```python
from build123d import *

# Parameters (mm, degrees)
SKETCH1_W           = 150
SKETCH1_H           = 150
SKETCH1_R           = 3
BOSS_EXTRUDE1_DEPTH = 60
SKETCH4_R           = 10
BOSS_EXTRUDE3_DEPTH = 8
SKETCH4_6_R         = 10
CUT_EXTRUDE1_DEPTH  = 5
SKETCH5_R           = 10
CUT_EXTRUDE2_DEPTH  = 5
SKETCH6_R           = 10
BOSS_EXTRUDE4_DEPTH = 5
SKETCH7_R           = 10
BOSS_EXTRUDE5_DEPTH = 5
CUT_EXTRUDE3_DEPTH  = 15


with BuildPart() as part:
    # Sketch1 → Boss-Extrude1 (new body)
    with BuildSketch(Plane(origin=(0, 0, 0), x_dir=(1, 0, 0), z_dir=(0, 1, 0))):
        with Locations((19.022617124, 32.835218094)):
            Rectangle(SKETCH1_W, SKETCH1_H)
        with Locations(Location((-43.477382875, 95.335218094, 0), (0, 0, 270))):
            Circle(SKETCH1_R, mode=Mode.SUBTRACT)
        with Locations(Location((-18.477382875, 95.335218094, 0), (0, 0, 270))):
            Circle(SKETCH1_R, mode=Mode.SUBTRACT)
        with Locations(Location((6.522617125, 95.335218094, 0), (0, 0, 270))):
            Circle(SKETCH1_R, mode=Mode.SUBTRACT)
        with Locations(Location((31.522617125, 95.335218094, 0), (0, 0, 270))):
            Circle(SKETCH1_R, mode=Mode.SUBTRACT)
        with Locations(Location((56.522617125, 95.335218094, 0), (0, 0, 270))):
            Circle(SKETCH1_R, mode=Mode.SUBTRACT)
        with Locations(Location((81.522617125, 95.335218094, 0), (0, 0, 270))):
            Circle(SKETCH1_R, mode=Mode.SUBTRACT)
        with Locations(Location((-18.477382875, 70.335218094, 0), (0, 0, 270))):
            Circle(SKETCH1_R, mode=Mode.SUBTRACT)
        with Locations(Location((6.522617125, 70.335218094, 0), (0, 0, 270))):
            Circle(SKETCH1_R, mode=Mode.SUBTRACT)
        with Locations(Location((31.522617125, 70.335218094, 0), (0, 0, 270))):
            Circle(SKETCH1_R, mode=Mode.SUBTRACT)
        with Locations(Location((56.522617125, 70.335218094, 0), (0, 0, 270))):
            Circle(SKETCH1_R, mode=Mode.SUBTRACT)
        with Locations(Location((81.522617125, 70.335218094, 0), (0, 0, 270))):
            Circle(SKETCH1_R, mode=Mode.SUBTRACT)
        with Locations(Location((-18.477382875, 45.335218094, 0), (0, 0, 270))):
            Circle(SKETCH1_R, mode=Mode.SUBTRACT)
        with Locations(Location((6.522617125, 45.335218094, 0), (0, 0, 270))):
            Circle(SKETCH1_R, mode=Mode.SUBTRACT)
        with Locations(Location((31.522617125, 45.335218094, 0), (0, 0, 270))):
            Circle(SKETCH1_R, mode=Mode.SUBTRACT)
        with Locations(Location((56.522617125, 45.335218094, 0), (0, 0, 270))):
            Circle(SKETCH1_R, mode=Mode.SUBTRACT)
        with Locations(Location((81.522617125, 45.335218094, 0), (0, 0, 270))):
            Circle(SKETCH1_R, mode=Mode.SUBTRACT)
        with Locations(Location((-18.477382875, 20.335218094, 0), (0, 0, 270))):
            Circle(SKETCH1_R, mode=Mode.SUBTRACT)
        with Locations(Location((6.522617125, 20.335218094, 0), (0, 0, 270))):
            Circle(SKETCH1_R, mode=Mode.SUBTRACT)
        with Locations(Location((31.522617125, 20.335218094, 0), (0, 0, 270))):
            Circle(SKETCH1_R, mode=Mode.SUBTRACT)
        with Locations(Location((56.522617125, 20.335218094, 0), (0, 0, 270))):
            Circle(SKETCH1_R, mode=Mode.SUBTRACT)
        with Locations(Location((81.522617125, 20.335218094, 0), (0, 0, 270))):
            Circle(SKETCH1_R, mode=Mode.SUBTRACT)
        with Locations(Location((-18.477382875, -4.664781906, 0), (0, 0, 270))):
            Circle(SKETCH1_R, mode=Mode.SUBTRACT)
        with Locations(Location((6.522617125, -4.664781906, 0), (0, 0, 270))):
            Circle(SKETCH1_R, mode=Mode.SUBTRACT)
        with Locations(Location((31.522617125, -4.664781906, 0), (0, 0, 270))):
            Circle(SKETCH1_R, mode=Mode.SUBTRACT)
        with Locations(Location((56.522617125, -4.664781906, 0), (0, 0, 270))):
            Circle(SKETCH1_R, mode=Mode.SUBTRACT)
        with Locations(Location((81.522617125, -4.664781906, 0), (0, 0, 270))):
            Circle(SKETCH1_R, mode=Mode.SUBTRACT)
        with Locations(Location((-18.477382875, -29.664781906, 0), (0, 0, 270))):
            Circle(SKETCH1_R, mode=Mode.SUBTRACT)
        with Locations(Location((6.522617125, -29.664781906, 0), (0, 0, 270))):
            Circle(SKETCH1_R, mode=Mode.SUBTRACT)
        with Locations(Location((31.522617125, -29.664781906, 0), (0, 0, 270))):
            Circle(SKETCH1_R, mode=Mode.SUBTRACT)
        with Locations(Location((56.522617125, -29.664781906, 0), (0, 0, 270))):
            Circle(SKETCH1_R, mode=Mode.SUBTRACT)
        with Locations(Location((81.522617125, -29.664781906, 0), (0, 0, 270))):
            Circle(SKETCH1_R, mode=Mode.SUBTRACT)
        with Locations(Location((-43.477382875, 70.335218094, 0), (0, 0, 270))):
            Circle(SKETCH1_R, mode=Mode.SUBTRACT)
        with Locations(Location((-43.477382875, 45.335218094, 0), (0, 0, 270))):
            Circle(SKETCH1_R, mode=Mode.SUBTRACT)
        with Locations(Location((-43.477382875, 20.335218094, 0), (0, 0, 270))):
            Circle(SKETCH1_R, mode=Mode.SUBTRACT)
        with Locations(Location((-43.477382875, -4.664781906, 0), (0, 0, 270))):
            Circle(SKETCH1_R, mode=Mode.SUBTRACT)
        with Locations(Location((-43.477382875, -29.664781906, 0), (0, 0, 270))):
            Circle(SKETCH1_R, mode=Mode.SUBTRACT)
    extrude(amount=BOSS_EXTRUDE1_DEPTH)

    # Sketch4 → Boss-Extrude3 (add)
    with BuildSketch(Plane(origin=(94.022617124, 0, 0), x_dir=(0, 0, -1), z_dir=(1, 0, 0))):
        with Locations((57.835218094, 30)):
            Circle(SKETCH4_R)
    extrude(amount=-BOSS_EXTRUDE3_DEPTH)

    # Sketch4_6 → Cut-Extrude1 (cut)
    with BuildSketch(Plane(origin=(94.022617124, 0, 0), x_dir=(0, 0, -1), z_dir=(1, 0, 0))):
        with Locations((7.835218094, 30)):
            Circle(SKETCH4_6_R)
        with Locations((57.835218094, 30)):
            Circle(SKETCH4_6_R)
    extrude(amount=-CUT_EXTRUDE1_DEPTH, mode=Mode.SUBTRACT)

    # Sketch5 → Cut-Extrude2 (cut)
    with BuildSketch(Plane(origin=(0, 0, -107.835218094), x_dir=(-1, 0, 0), z_dir=(0, 0, -1))):
        with Locations((-44.022617124, 30)):
            Circle(SKETCH5_R)
        with Locations((5.977382876, 30)):
            Circle(SKETCH5_R)
    extrude(amount=-CUT_EXTRUDE2_DEPTH, mode=Mode.SUBTRACT)

    # Sketch6 → Boss-Extrude4 (add)
    with BuildSketch(Plane.ZY.offset(55.977382876)):
        with Locations(Location((-57.835218094, 30, 0), (0, 0, 180))):
            Circle(SKETCH6_R)
        with Locations(Location((-7.835218094, 30, 0), (0, 0, 180))):
            Circle(SKETCH6_R)
    extrude(amount=BOSS_EXTRUDE4_DEPTH)

    # Sketch7 → Boss-Extrude5 (add)
    with BuildSketch(Plane.XY.offset(42.164781906)):
        with Locations(Location((-5.977382876, 30, 0), (0, 0, 180))):
            Circle(SKETCH7_R)
        with Locations(Location((44.022617124, 30, 0), (0, 0, 180))):
            Circle(SKETCH7_R)
    extrude(amount=BOSS_EXTRUDE5_DEPTH)

    # Sketch8 → Cut-Extrude3 (cut)
    with BuildSketch(Plane.XZ):
        with BuildLine():
            Line((-41.977382876, 38.164781906), (80.022617124, 38.164781906))
            ThreePointArc((80.022617124, 38.164781906), (87.093684936, 35.235849718), (90.022617124, 28.164781906))
            Line((90.022617124, 28.164781906), (90.022617124, -93.835218094))
            ThreePointArc((90.022617124, -93.835218094), (87.093684936, -100.906285906), (80.022617124, -103.835218094))
            Line((80.022617124, -103.835218094), (-41.977382876, -103.835218094))
            ThreePointArc((-41.977382876, -103.835218094), (-49.048450687, -100.906285906), (-51.977382876, -93.835218094))
            Line((-51.977382876, -93.835218094), (-51.977382876, 28.164781906))
            ThreePointArc((-51.977382876, 28.164781906), (-49.048450687, 35.235849718), (-41.977382876, 38.164781906))
        make_face()
    extrude(amount=-CUT_EXTRUDE3_DEPTH, mode=Mode.SUBTRACT)


solid = part.part
```
Check sheet for the modelled part. Datum: model origin and axes. Units: mm. A direction names the side the tool comes from. Coordinates: 2 decimals unless noted, no trailing zeros. Order: outer loops, then holes, each group sorted by start corner. A loop starts at its lowest first (then second) coordinate and runs counter-clockwise, first axis right, second up. Notation, with made-up numbers: M 15.5,37 L 39.5,37 A23 cw 39.5,72 Z; hole C -25,-11 d7. An arc over 180 degrees is marked long. One line per question, with ' | ' between items. Start each with the question number.
Item 1: Sectioned sample at A-A on y = 7.5. Record the cut outline in (x, z), and give its area (3 significant figures).
Item 2: Sectioned sample at B-B on z = -35. Record the cut outline in (x, y), and give its area (3 significant figures).
Item 3: Mould release check, pull along X, two halves, no side actions. Record for faces 4 (the cylindrical face through (4.7, 37.18, -72.72)), 5 (the cylindrical face through (-40.95, 37.18, 31.28)), 6 (the flat face through (89.023, 30, -8)), 7 (the cylindrical face through (91.56, 21.13, -12.45)): pulls with the +X half, pulls with the -X half, needs draft (parallel to the pull), parting line crosses it, or undercut.
Item 4: Access from +Z, -Z, +X, -X, +Y, -Y to the whole of each face (thin tool, end or side, straight path). Record for faces 1 (the flat face through (18, 7, 38.165)), 2 (the cylindrical face through (-15.5, 37.2, 4.3)), 3 (the flat face through (44, 30, -102.835)).
Item 5: Sectioned sample at C-C on x = 22. Record the cut outline in (y, z), and give its area (3 significant figures).
Item 6: Material ranges on line 1 (X direction, y = 3, z = -77.5); line 2 (X direction, y = 45, z = 23); line 3 (Y direction, x = -41, z = 14), recorded low to high.
Item 7: Sectioned sample at D-D on z = 5. Count the separate pieces of the cut face and the enclosed holes in it, and give its area (3 significant figures).
Item 8: Gauge pin test, flat ends, axial feed: P1, Ø8, axis at x = 6.52, z = -70.34, coming from the -Y side; P2, Ø1.5, axis at x = 28.5, y = 10, coming from the +Z side; P3, Ø4, axis at y = 20.5, z = 6.5, coming from the -X side. Record the tip position at first contact, or that the pin passes through.
Answer below:
1) outline: M -55.98,-107.84 L 94.02,-107.84 L 94.02,42.16 L -55.98,42.16 Z; hole M -51.98,-93.84 A10 ccw -41.98,-103.84 L 80.02,-103.84 A10 ccw 90.02,-93.84 L 90.02,28.16 A10 ccw 80.02,38.16 L -41.98,38.16 A10 ccw -51.98,28.16 Z | area: 2,420 mm^2
2) outline: M -55.98,0 L -51.98,0 L -51.98,15 L 90.02,15 L 90.02,0 L 94.02,0 L 94.02,60 L -55.98,60 Z | area: 6,870 mm^2
3) face 4: undercut | face 5: undercut | face 6: pulls with the +X half | face 7: needs draft
4) face 1: -Y | face 2: +Y, -Y | face 3: -Z
5) outline: M 0,-107.84 L 60,-107.84 L 60,42.16 L 0,42.16 L 0,38.16 L 15,38.16 L 15,-103.84 L 0,-103.84 Z | area: 6,870 mm^2
6) line 1: x = -55.98 to -51.98, 90.02 to 94.02 | line 2: x = -55.98 to 94.02 | line 3: y = 15 to 60
7) separate pieces: 7 | enclosed holes: 0 | area: 5,260 mm^2
8) P1: stops at y = 15 | P2: stops at z = 42.16 | P3: stops at x = -55.98
